from build123d import *

# Parameters (mm, degrees)
SKETCH_1_R               = 12.5
SKETCH_1_R_2             = 4
SKETCH_1_R_3             = 2.5
EXTRUDE_1_DEPTH          = 7.8
SKETCH_1_3_R             = 3.1
SKETCH_1_3_R_2           = 2.5
CUT_EXTRUDE_1_DEPTH      = 1.5
CUT_EXTRUDE_START        = 6.3
SKETCH_1_4_R             = 3.1
SKETCH_1_4_R_2           = 2.5
CUT_EXTRUDE_2_DEPTH      = 1.5
SKETCH_2_R               = 18.5
SKETCH_2_R_2             = 12.5
EXTRUDE_2_DEPTH          = 4
SKETCH_2_3_R             = 18.5
SKETCH_2_3_R_2           = 16.5
EXTRUDE_3_DEPTH          = 11
EXTRUDE_START            = 63
EXTRUDE_4_DEPTH          = 52
CUT_EXTRUDE_3_DEPTH      = 69.216566903
CUT_EXTRUDE_3_DEPTH_BACK = 69.216566903
SKETCH_5_R               = 0.75


with BuildPart() as part:
    # Sketch 1 → Extrude 1 (new body)
    with BuildSketch(Plane(origin=(0, 0, 0), x_dir=(0, 0, -1), z_dir=(1, 0, 0))):
        Circle(SKETCH_1_R)
        Circle(SKETCH_1_R_2, mode=Mode.SUBTRACT)
        with Locations((0, 8)):
            Circle(SKETCH_1_R_3, mode=Mode.SUBTRACT)
        with Locations((8, 0)):
            Circle(SKETCH_1_R_3, mode=Mode.SUBTRACT)
        with Locations((0, -8)):
            Circle(SKETCH_1_R_3, mode=Mode.SUBTRACT)
        with Locations((-8, 0)):
            Circle(SKETCH_1_R_3, mode=Mode.SUBTRACT)
    extrude(amount=EXTRUDE_1_DEPTH)

    # Sketch 1_3 → Cut-Extrude 1 (cut)
    # profile 1 of 4: a face of its own
    with BuildSketch(Plane(origin=(0, 0, 0), x_dir=(0, 0, -1), z_dir=(1, 0, 0))):
        with Locations((0, 8)):
            Circle(SKETCH_1_3_R)
        with Locations((0, 8)):
            Circle(SKETCH_1_3_R_2, mode=Mode.SUBTRACT)
    # profile 2 of 4: a face of its own
    with BuildSketch(Plane(origin=(0, 0, 0), x_dir=(0, 0, -1), z_dir=(1, 0, 0))):
        with Locations((8, 0)):
            Circle(SKETCH_1_3_R)
        with Locations((8, 0)):
            Circle(SKETCH_1_3_R_2, mode=Mode.SUBTRACT)
    # profile 3 of 4: a face of its own
    with BuildSketch(Plane(origin=(0, 0, 0), x_dir=(0, 0, -1), z_dir=(1, 0, 0))):
        with Locations((0, -8)):
            Circle(SKETCH_1_3_R)
        with Locations((0, -8)):
            Circle(SKETCH_1_3_R_2, mode=Mode.SUBTRACT)
    # profile 4 of 4: a face of its own
    with BuildSketch(Plane(origin=(0, 0, 0), x_dir=(0, 0, -1), z_dir=(1, 0, 0))):
        with Locations((-8, 0)):
            Circle(SKETCH_1_3_R)
        with Locations((-8, 0)):
            Circle(SKETCH_1_3_R_2, mode=Mode.SUBTRACT)
    extrude(amount=CUT_EXTRUDE_1_DEPTH, mode=Mode.SUBTRACT)

    # Sketch 1_4 → Cut-Extrude 2 (cut)
    # profile 1 of 4: a face of its own
    with BuildSketch(Plane(origin=(0, 0, 0), x_dir=(0, 0, -1), z_dir=(1, 0, 0)).offset(CUT_EXTRUDE_START)):
        with Locations((0, 8)):
            Circle(SKETCH_1_4_R)
        with Locations((0, 8)):
            Circle(SKETCH_1_4_R_2, mode=Mode.SUBTRACT)
    # profile 2 of 4: a face of its own
    with BuildSketch(Plane(origin=(0, 0, 0), x_dir=(0, 0, -1), z_dir=(1, 0, 0)).offset(CUT_EXTRUDE_START)):
        with Locations((8, 0)):
            Circle(SKETCH_1_4_R)
        with Locations((8, 0)):
            Circle(SKETCH_1_4_R_2, mode=Mode.SUBTRACT)
    # profile 3 of 4: a face of its own
    with BuildSketch(Plane(origin=(0, 0, 0), x_dir=(0, 0, -1), z_dir=(1, 0, 0)).offset(CUT_EXTRUDE_START)):
        with Locations((0, -8)):
            Circle(SKETCH_1_4_R)
        with Locations((0, -8)):
            Circle(SKETCH_1_4_R_2, mode=Mode.SUBTRACT)
    # profile 4 of 4: a face of its own
    with BuildSketch(Plane(origin=(0, 0, 0), x_dir=(0, 0, -1), z_dir=(1, 0, 0)).offset(CUT_EXTRUDE_START)):
        with Locations((-8, 0)):
            Circle(SKETCH_1_4_R)
        with Locations((-8, 0)):
            Circle(SKETCH_1_4_R_2, mode=Mode.SUBTRACT)
    extrude(amount=CUT_EXTRUDE_2_DEPTH, mode=Mode.SUBTRACT)



with BuildPart() as body_2:
    # Sketch 2 → Extrude 2 (new body)
    with BuildSketch(Plane.ZY):
        Circle(SKETCH_2_R)
        with Locations(Location((0, 0, 0), (0, 0, 180))):
            Circle(SKETCH_2_R_2, mode=Mode.SUBTRACT)
    extrude(amount=-EXTRUDE_2_DEPTH)


with BuildPart() as part_1:
    add(part.part)

    add(body_2.part)  # Extrude 3 merges body 2
    # Sketch 2_3 → Extrude 3 (add)
    with BuildSketch(Plane.ZY):
        Circle(SKETCH_2_3_R)
        Circle(SKETCH_2_3_R_2, mode=Mode.SUBTRACT)
    extrude(amount=EXTRUDE_3_DEPTH)

    # Sketch 2_4 → Extrude 4 (add)
    with BuildSketch(Plane.ZY.offset(EXTRUDE_START)):
        with BuildLine():
            ThreePointArc((-4, -18.062391868), (-2.011933204, -18.390272559), (0, -18.5))
            ThreePointArc((0, -18.5), (2.011933204, -18.390272559), (4, -18.062391868))
            Line((4, -18.062391868), (4, -16.007810594))
            ThreePointArc((4, -16.007810594), (0, -16.5), (-4, -16.007810594))
            Line((-4, -16.007810594), (-4, -18.062391868))
        make_face()
        with BuildLine():
            ThreePointArc((0, 18.5), (-2.011933204, 18.390272559), (-4, 18.062391868))
            Line((-4, 18.062391868), (-4, 16.007810594))
            ThreePointArc((-4, 16.007810594), (0, 16.5), (4, 16.007810594))
            Line((4, 16.007810594), (4, 18.062391868))
            ThreePointArc((4, 18.062391868), (2.011933204, 18.390272559), (0, 18.5))
        make_face()
    extrude(amount=-EXTRUDE_4_DEPTH)

    # Sketch 5 → Cut-Extrude 3 (cut, two sides: drawn at the far end of the back side and taken through both)
    with BuildSketch(Plane(origin=(0, 0, 0), x_dir=(1, 0, 0), z_dir=(0, 1, 0)).offset(-CUT_EXTRUDE_3_DEPTH_BACK)):
        with Locations(Location((-59.5, 0, 0), (0, 0, 270))):
            Circle(SKETCH_5_R)
        with Locations(Location((-30.3, 0, 0), (0, 0, 270))):
            Circle(SKETCH_5_R)
    extrude(amount=CUT_EXTRUDE_3_DEPTH + CUT_EXTRUDE_3_DEPTH_BACK, mode=Mode.SUBTRACT)


solid = part_1.part
Read the model definition and answer for the solid it produces. Units are mm, in the model's axes. A direction names the side the tool comes from. Round coordinates to 2 decimals unless told otherwise and drop trailing zeros. Order: outer loops, then holes, each group sorted by start corner. A loop starts at its lowest first (then second) coordinate and runs counter-clockwise, first axis right, second up.
1) The part is cut by section B-B on z = 8. Write down the section's boundary in (x, y).
2) Straight lines are drawn through the part: L1, parallel to Z at x = -5.75, y = 0; L2, parallel to X at y = 11, z = -10.5. For each, find the intervals that lie inside material, in ascending order.
3) For faces 1 (the face through (0.7, 0.1, -4.9)), 2 (the face through (-63, 17, 0)), 3 (the face through (-37, -17, 4)), 4 (the face through (3.87, -10.44, 0.54)), 5 (the face through (7.04, -4.926, 0.404)), determine the directions among +Z, -Z, +X, -X, +Y, -Y from which every point of the face is accessible in a straight line to the end or side of a thin tool.
4) The part is cut by section A-A on x = 3. Write down the section's boundary in (y, z).
5) The mould has two halves that part along X. Classify faces 6 (the face through (-58.756, -17.506, -0.098)), 7 (the face through (7.8, 3, 3)), 8 (the face through (3.9, 0.1, 10.5)): released by +X, released by -X, zero draft, split by the parting line, or undercut.
6) The part is cut by section C-C on x = -26. Write down the section's boundary in (y, z), plus the area to 3 significant figures.
7) Flat-ended cylindrical pins translate along their axes: pin 1 (7.5 mm diameter, centred on y = 2, z = 9, fed in from -X); pin 2 (5 mm diameter, centred on y = 0, z = 0, fed in from +X); pin 3 (16 mm diameter, centred on y = -4.5, z = -14, fed in from -X); pin 4 (3 mm diameter, centred on y = -7, z = 0.5, fed in from -X). Find the tip coordinate at first contact, or state that the pin passes through.
Resolved:
1. outline: (-11, -16.68) - (4, -16.68) - (4, -9.6) - (7.8, -9.6) - (7.8, -3.1) - (6.3, -3.1) - (6.3, -2.5) - (1.5, -2.5) - (1.5, -3.1) - (0, -3.1) - (0, -14.43) - (-11, -14.43) - close; (-11, 14.43) - (0, 14.43) - (0, 3.1) - (1.5, 3.1) - (1.5, 2.5) - (6.3, 2.5) - (6.3, 3.1) - (7.8, 3.1) - (7.8, 9.6) - (4, 9.6) - (4, 16.68) - (-11, 16.68) - close
2. L1: z = -18.5 to -16.5, 16.5 to 18.5
2. L2: x = 0 to 4
3. face 1: -X
3. face 2: +Z, -Z, -X, +Y, -Y
3. face 3: +Z, -X, +Y, -Y
3. face 4: +X, -X
3. face 5: +X
4. outline: circle Ø37 at (0, 0); hole circle Ø5 at (-8, 0); hole circle Ø8 at (0, 0); hole circle Ø5 at (0, -8); hole circle Ø5 at (0, 8); hole circle Ø5 at (8, 0)
5. face 6: undercut
5. face 7: released by +X
5. face 8: zero draft
6. outline: (-18.06, -4) - (-16.01, -4) arc R16.5 cw to (-16.01, 4) - (-18.06, 4) arc R18.5 ccw to start; (16.01, -4) - (18.06, -4) arc R18.5 ccw to (18.06, 4) - (16.01, 4) arc R16.5 cw to start
6. area: 32.3 mm2
7. pin 1: stops at x = 0
7. pin 2: passes through
7. pin 3: stops at x = -11
7. pin 4: stops at x = 1.5
